```python
from build123d import *

# Parameters (mm, degrees)
F1_DEPTH = 7.8
F0_R     = 7.25
F2_DEPTH = 1.9
F3_SIZE  = 1
F4_R     = 0.7


# Not quite as in the source:
# - a feature names something its author has since deleted; it is built from what else it names


with BuildPart() as f1:
    # F0 (on Top) → F1 (new body)
    with BuildSketch(Plane.XY):
        with BuildLine():
            ThreePointArc((1.8904761229, -0.1900000758), (0, -1.9), (-1.8904761229, -0.1900000758))
            Line((-1.8904761229, -0.1900000758), (-3.1192186475, -0.1900000758))
            ThreePointArc((-3.1192186475, -0.1900000758), (0, -3.125), (3.1192186475, -0.1900000758))
            Line((3.1192186475, -0.1900000758), (1.8904761229, -0.1900000758))
        make_face()
        with BuildLine():
            ThreePointArc((-1.8904761229, -0.1900000758), (-0.0951193107, 1.897617537), (1.9, 0))
            ThreePointArc((1.9, 0), (1.897617537, -0.0951193107), (1.8904761229, -0.1900000758))
            Line((1.8904761229, -0.1900000758), (3.1192186475, -0.1900000758))
            ThreePointArc((3.1192186475, -0.1900000758), (3.1235543275, -0.0950440067), (3.125, 0))
            ThreePointArc((3.125, 0), (-0.0950440067, 3.1235543275), (-3.1192186475, -0.1900000758))
            Line((-3.1192186475, -0.1900000758), (-1.8904761229, -0.1900000758))
        make_face()
    extrude(amount=-F1_DEPTH)

    # F0 (on Top) → F2 (join)
    with BuildSketch(Plane.XY):
        with Locations((2.98e-08, -1.6900000758)):
            Circle(F0_R)
        Polygon((2.5797043927, -5.2021308802), (0, -7.9360147938), (-2.5797043927, -5.2021308802), align=None, mode=Mode.SUBTRACT)
        with BuildLine():
            Line((-5.4999999702, -0.1900000758), (-3.1192186475, -0.1900000758))
            ThreePointArc((-3.1192186475, -0.1900000758), (-0.0950440067, 3.1235543275), (3.125, 0))
            ThreePointArc((3.125, 0), (3.1235543275, -0.0950440067), (3.1192186475, -0.1900000758))
            Line((3.1192186475, -0.1900000758), (5.5000000298, -0.1900000758))
            Line((5.5000000298, -0.1900000758), (5.5000000298, -3.1900000758))
            Line((5.5000000298, -3.1900000758), (-5.4999999702, -3.1900000758))
            Line((-5.4999999702, -3.1900000758), (-5.4999999702, -0.1900000758))
        make_face(mode=Mode.SUBTRACT)
        with BuildLine():
            ThreePointArc((3.1192186475, -0.1900000758), (0, -3.125), (-3.1192186475, -0.1900000758))
            Line((-3.1192186475, -0.1900000758), (-5.4999999702, -0.1900000758))
            Line((-5.4999999702, -0.1900000758), (-5.4999999702, -3.1900000758))
            Line((-5.4999999702, -3.1900000758), (5.5000000298, -3.1900000758))
            Line((5.5000000298, -3.1900000758), (5.5000000298, -0.1900000758))
            Line((5.5000000298, -0.1900000758), (3.1192186475, -0.1900000758))
        make_face()
        with BuildLine():
            ThreePointArc((-1.8904761229, -0.1900000758), (-0.0951193107, 1.897617537), (1.9, 0))
            ThreePointArc((1.9, 0), (1.897617537, -0.0951193107), (1.8904761229, -0.1900000758))
            Line((1.8904761229, -0.1900000758), (3.1192186475, -0.1900000758))
            ThreePointArc((3.1192186475, -0.1900000758), (3.1235543275, -0.0950440067), (3.125, 0))
            ThreePointArc((3.125, 0), (-0.0950440067, 3.1235543275), (-3.1192186475, -0.1900000758))
            Line((-3.1192186475, -0.1900000758), (-1.8904761229, -0.1900000758))
        make_face()
        with BuildLine():
            ThreePointArc((1.8904761229, -0.1900000758), (0, -1.9), (-1.8904761229, -0.1900000758))
            Line((-1.8904761229, -0.1900000758), (-3.1192186475, -0.1900000758))
            ThreePointArc((-3.1192186475, -0.1900000758), (0, -3.125), (3.1192186475, -0.1900000758))
            Line((3.1192186475, -0.1900000758), (1.8904761229, -0.1900000758))
        make_face()
        Polygon((-2.5797043927, -5.2021308802), (0, -7.9360147938), (2.5797043927, -5.2021308802), align=None)
        with BuildLine():
            ThreePointArc((1.8904761229, -0.1900000758), (1.897617537, -0.0951193107), (1.9, 0))
            ThreePointArc((1.9, 0), (-0.0951193107, 1.897617537), (-1.8904761229, -0.1900000758))
            Line((-1.8904761229, -0.1900000758), (1.8904761229, -0.1900000758))
        make_face()
        with BuildLine():
            Line((1.8904761229, -0.1900000758), (-1.8904761229, -0.1900000758))
            ThreePointArc((-1.8904761229, -0.1900000758), (0, -1.9), (1.8904761229, -0.1900000758))
        make_face()
    extrude(amount=F2_DEPTH)

    # F3
    f3_edges = [f1.edges().sort_by_distance(p)[0] for p in [
        (3.119219, 0.19, -7.8),
    ]]
    chamfer(f3_edges, length=F3_SIZE)

    # F4
    f4_edges = [f1.edges().sort_by_distance(p)[0] for p in [
        (-7.25, -1.69, 0),
        (-7.25, -1.69, 1.9),
    ]]
    fillet(f4_edges, radius=F4_R)


solid = f1.part
```
Work out the finished part from the listing and answer in its coordinate system (mm). Give positions to 0.01 mm unless a question says otherwise; leave off trailing zeros. Loops run counter-clockwise (first coordinate to the right, second up) from the corner with the lowest first, then second, coordinate; pieces in that order, holes last. Notation, with made-up numbers: (-37, -20.5) -> (10, -20.5) arc R22 cw to (10, 9.5) -> close; hole circle Ø5 at (79.25, 38.5). An arc over 180 degrees is marked (long way). One line per question, with ' | ' between items. Start each with the question number.
1) Section A-A, the plane z = -1.75 is taken. Determine the outline of the cut face in (x, y) (3 decimals), then the cut area to 3 significant figures.
2) Section B-B, the plane z = 1 is taken. Determine the outline of the cut face in (x, y).
3) Each of these flat-tipped pins is pushed along its axis until it touches: pin 1 (1.5 mm diameter, centred on y = -0.5, z = 0.5, fed in from +X); pin 2 (3 mm diameter, centred on y = 0.5, z = -6, fed in from -X) (3 decimals); pin 3 (1.5 mm diameter, centred on x = 1.5, z = -6, fed in from +Y). Where does it stop, or does it pass through?
4) Determine the mould class of faces 1 (the face through (-5.753, -6.102, 0.946)), 2 (the face through (0, -2, 1.9)), 3 (the face through (0, 0, 0)) for opening direction X: +X half, -X half, draft (parallel to the pull), parting line (faces both ways), or undercut.
5) Straight lines are drawn through the part: L1, parallel to Z at x = 2.75, y = -7; L2, parallel to Y at x = 1, z = -1.25; L3, parallel to Y at x = 1.5, z = -1. For each, find the intervals that lie inside material, in ascending order.
Resolved:
1) outline: circle Ø6.25 at (0, 0); hole circle Ø3.8 at (0, 0) | area: 19.3 mm2
2) outline: circle Ø14.5 at (0, -1.69)
3) pin 1: x = 7.24 | pin 2: x = -3.125 | pin 3: y = 3.03
4) face 1: parting line | face 2: draft | face 3: undercut
5) L1: 0 to 1.9 | L2: -2.96 to -1.62, 1.62 to 2.96 | L3: -2.74 to -1.17, 1.17 to 2.74
